Geometry check sheet. Reference: the model listing, model coordinates, mm. Round coordinates to 2 decimals unless told otherwise and drop trailing zeros. Write each loop counter-clockwise with the first axis right and the second up, starting at its lowest first coordinate (ties: lowest second). Pieces come first, ordered by that corner, then holes.
Item 1: Cross-section at A-A (x = -100). Enter the section's corners in (y, z).
Item 2: Draft check along X on faces 1 (the face through (-45, 2, 25)), 2 (the face through (150, 2, -1)), 3 (the face through (2, 5, -11)). Enter one of: pulls with the +X half, pulls with the -X half, needs draft (parallel to the pull), parting line crosses it, or undercut.
Item 3: Cross-section at C-C (x = 18). Enter the section's corners in (y, z), then the cut area to 3 significant figures.
Item 4: Cross-section at B-B (y = 3.05). State how many separate pieces and enclosed holes the cut face has, then the cut area to 3 significant figures.
Item 5: Scan lines: probe 1 along Z at (x, y) = (92, 1.8); probe 2 along Z at (x, y) = (138.25, 3.35); probe 3 along X at (y, z) = (0.9, -28). Record each from-to range of solid material in increasing order.
Item 6: Depth check by flat-ended pin: P1, Ø9, axis at x = 0, z = 0, coming from the +Y side. Enter the tip coordinate at first touch or a pass-through.
from build123d import *

# Parameters (mm, degrees)
SKETCH1_R           = 7.5
SKETCH1_R_2         = 1.75
SKETCH1_W           = 5
SKETCH1_H           = 10
BOSS_EXTRUDE2_DEPTH = 5


with BuildPart() as part:
    # Sketch1 → Boss-Extrude2 (new body)
    with BuildSketch(Plane(origin=(0, 0, 0), x_dir=(1, 0, 0), z_dir=(0, 1, 0))):
        Polygon((-50, 45), (150, 45), (150, -45), (-50, -45), (-150, -45), (-150, 45), align=None)
        Circle(SKETCH1_R, mode=Mode.SUBTRACT)
        with Locations((100, 0)):
            Circle(SKETCH1_R, mode=Mode.SUBTRACT)
        with Locations((-100, 0)):
            Circle(SKETCH1_R, mode=Mode.SUBTRACT)
        with Locations((-138.25, 25)):
            Circle(SKETCH1_R_2, mode=Mode.SUBTRACT)
        with Locations((-130, 38.25)):
            Circle(SKETCH1_R_2, mode=Mode.SUBTRACT)
        with Locations((-138.25, -25)):
            Circle(SKETCH1_R_2, mode=Mode.SUBTRACT)
        with Locations((-70, 38.25)):
            Circle(SKETCH1_R_2, mode=Mode.SUBTRACT)
        with Locations((-30, 38.25)):
            Circle(SKETCH1_R_2, mode=Mode.SUBTRACT)
        with Locations((30, 38.25)):
            Circle(SKETCH1_R_2, mode=Mode.SUBTRACT)
        with Locations((70, 38.25)):
            Circle(SKETCH1_R_2, mode=Mode.SUBTRACT)
        with Locations((130, 38.25)):
            Circle(SKETCH1_R_2, mode=Mode.SUBTRACT)
        with Locations((-130, -38.25)):
            Circle(SKETCH1_R_2, mode=Mode.SUBTRACT)
        with Locations((-70, -38.25)):
            Circle(SKETCH1_R_2, mode=Mode.SUBTRACT)
        with Locations((-30, -38.25)):
            Circle(SKETCH1_R_2, mode=Mode.SUBTRACT)
        with Locations((30, -38.25)):
            Circle(SKETCH1_R_2, mode=Mode.SUBTRACT)
        with Locations((70, -38.25)):
            Circle(SKETCH1_R_2, mode=Mode.SUBTRACT)
        with Locations((130, -38.25)):
            Circle(SKETCH1_R_2, mode=Mode.SUBTRACT)
        with Locations((138.25, -25)):
            Circle(SKETCH1_R_2, mode=Mode.SUBTRACT)
        with Locations((138.25, 25)):
            Circle(SKETCH1_R_2, mode=Mode.SUBTRACT)
        with BuildLine():
            Line((-21.910531466, 30), (21.910531466, 30))
            ThreePointArc((21.910531466, 30), (23.786301496, 28.693892495), (23.212114213, 26.481486795))
            Line((23.212114213, 26.481486795), (8.508395839, 13.878299617))
            ThreePointArc((8.508395839, 13.878299617), (7.476831919, 13.41512419), (6.358952728, 13.585423078))
            ThreePointArc((6.358952728, 13.585423078), (0, 15), (-6.358952728, 13.585423078))
            ThreePointArc((-6.358952728, 13.585423078), (-7.476831919, 13.41512419), (-8.508395839, 13.878299617))
            Line((-8.508395839, 13.878299617), (-23.212114213, 26.481486795))
            ThreePointArc((-23.212114213, 26.481486795), (-23.786301496, 28.693892495), (-21.910531466, 30))
        make_face(mode=Mode.SUBTRACT)
        with BuildLine():
            Line((-35, 19.066169828), (-35, -19.066169828))
            ThreePointArc((-35, -19.066169828), (-33.835713619, -20.883195625), (-31.698417253, -20.584683033))
            Line((-31.698417253, -20.584683033), (-15.016309573, -6.285733593))
            ThreePointArc((-15.016309573, -6.285733593), (-14.400814669, -5.337144314), (-14.398140282, -4.206370931))
            ThreePointArc((-14.398140282, -4.206370931), (-15, 0), (-14.398140282, 4.206370931))
            ThreePointArc((-14.398140282, 4.206370931), (-14.400814669, 5.337144314), (-15.016309573, 6.285733593))
            Line((-15.016309573, 6.285733593), (-31.698417253, 20.584683033))
            ThreePointArc((-31.698417253, 20.584683033), (-33.835713619, 20.883195625), (-35, 19.066169828))
        make_face(mode=Mode.SUBTRACT)
        with BuildLine():
            Line((-21.910531466, -30), (21.910531466, -30))
            ThreePointArc((21.910531466, -30), (23.786301496, -28.693892495), (23.212114213, -26.481486795))
            Line((23.212114213, -26.481486795), (8.508395839, -13.878299617))
            ThreePointArc((8.508395839, -13.878299617), (7.476831919, -13.41512419), (6.358952728, -13.585423078))
            ThreePointArc((6.358952728, -13.585423078), (0, -15), (-6.358952728, -13.585423078))
            ThreePointArc((-6.358952728, -13.585423078), (-7.476831919, -13.41512419), (-8.508395839, -13.878299617))
            Line((-8.508395839, -13.878299617), (-23.212114213, -26.481486795))
            ThreePointArc((-23.212114213, -26.481486795), (-23.786301496, -28.693892495), (-21.910531466, -30))
        make_face(mode=Mode.SUBTRACT)
        with BuildLine():
            Line((35, 19.066169828), (35, -19.066169828))
            ThreePointArc((35, -19.066169828), (33.835713619, -20.883195625), (31.698417253, -20.584683033))
            Line((31.698417253, -20.584683033), (15.016309573, -6.285733593))
            ThreePointArc((15.016309573, -6.285733593), (14.400814669, -5.337144314), (14.398140282, -4.206370931))
            ThreePointArc((14.398140282, -4.206370931), (15, 0), (14.398140282, 4.206370931))
            ThreePointArc((14.398140282, 4.206370931), (14.400814669, 5.337144314), (15.016309573, 6.285733593))
            Line((15.016309573, 6.285733593), (31.698417253, 20.584683033))
            ThreePointArc((31.698417253, 20.584683033), (33.835713619, 20.883195625), (35, 19.066169828))
        make_face(mode=Mode.SUBTRACT)
        with BuildLine():
            Line((131.698417253, -20.584683033), (115.016309573, -6.285733593))
            ThreePointArc((115.016309573, -6.285733593), (114.400814669, -5.337144314), (114.398140282, -4.206370931))
            ThreePointArc((114.398140282, -4.206370931), (115, 0), (114.398140282, 4.206370931))
            ThreePointArc((114.398140282, 4.206370931), (114.400814669, 5.337144314), (115.016309573, 6.285733593))
            Line((115.016309573, 6.285733593), (131.698417253, 20.584683033))
            ThreePointArc((131.698417253, 20.584683033), (133.835713619, 20.883195625), (135, 19.066169828))
            Line((135, 19.066169828), (135, -19.066169828))
            ThreePointArc((135, -19.066169828), (133.835713619, -20.883195625), (131.698417253, -20.584683033))
        make_face(mode=Mode.SUBTRACT)
        with BuildLine():
            Line((123.212114213, -26.481486795), (108.508395839, -13.878299617))
            ThreePointArc((108.508395839, -13.878299617), (107.476831919, -13.41512419), (106.358952728, -13.585423078))
            ThreePointArc((106.358952728, -13.585423078), (100, -15), (93.641047272, -13.585423078))
            ThreePointArc((93.641047272, -13.585423078), (92.523168081, -13.41512419), (91.491604161, -13.878299617))
            Line((91.491604161, -13.878299617), (76.787885787, -26.481486795))
            ThreePointArc((76.787885787, -26.481486795), (76.213698504, -28.693892495), (78.089468534, -30))
            Line((78.089468534, -30), (121.910531466, -30))
            ThreePointArc((121.910531466, -30), (123.786301496, -28.693892495), (123.212114213, -26.481486795))
        make_face(mode=Mode.SUBTRACT)
        with BuildLine():
            Line((68.301582747, -20.584683033), (84.983690427, -6.285733593))
            ThreePointArc((84.983690427, -6.285733593), (85.599185331, -5.337144314), (85.601859718, -4.206370931))
            ThreePointArc((85.601859718, -4.206370931), (85, 0), (85.601859718, 4.206370931))
            ThreePointArc((85.601859718, 4.206370931), (85.599185331, 5.337144314), (84.983690427, 6.285733593))
            Line((84.983690427, 6.285733593), (68.301582747, 20.584683033))
            ThreePointArc((68.301582747, 20.584683033), (66.164286381, 20.883195625), (65, 19.066169828))
            Line((65, 19.066169828), (65, -19.066169828))
            ThreePointArc((65, -19.066169828), (66.164286381, -20.883195625), (68.301582747, -20.584683033))
        make_face(mode=Mode.SUBTRACT)
        with BuildLine():
            Line((76.787885787, 26.481486795), (91.491604161, 13.878299617))
            ThreePointArc((91.491604161, 13.878299617), (92.523168081, 13.41512419), (93.641047272, 13.585423078))
            ThreePointArc((93.641047272, 13.585423078), (100, 15), (106.358952728, 13.585423078))
            ThreePointArc((106.358952728, 13.585423078), (107.476831919, 13.41512419), (108.508395839, 13.878299617))
            Line((108.508395839, 13.878299617), (123.212114213, 26.481486795))
            ThreePointArc((123.212114213, 26.481486795), (123.786301496, 28.693892495), (121.910531466, 30))
            Line((121.910531466, 30), (78.089468534, 30))
            ThreePointArc((78.089468534, 30), (76.213698504, 28.693892495), (76.787885787, 26.481486795))
        make_face(mode=Mode.SUBTRACT)
        with BuildLine():
            Line((-68.301582747, -20.584683033), (-84.983690427, -6.285733593))
            ThreePointArc((-84.983690427, -6.285733593), (-85.599185331, -5.337144314), (-85.601859718, -4.206370931))
            ThreePointArc((-85.601859718, -4.206370931), (-85, 0), (-85.601859718, 4.206370931))
            ThreePointArc((-85.601859718, 4.206370931), (-85.599185331, 5.337144314), (-84.983690427, 6.285733593))
            Line((-84.983690427, 6.285733593), (-68.301582747, 20.584683033))
            ThreePointArc((-68.301582747, 20.584683033), (-66.164286381, 20.883195625), (-65, 19.066169828))
            Line((-65, 19.066169828), (-65, -19.066169828))
            ThreePointArc((-65, -19.066169828), (-66.164286381, -20.883195625), (-68.301582747, -20.584683033))
        make_face(mode=Mode.SUBTRACT)
        with BuildLine():
            Line((-76.787885787, -26.481486795), (-91.491604161, -13.878299617))
            ThreePointArc((-91.491604161, -13.878299617), (-92.523168081, -13.41512419), (-93.641047272, -13.585423078))
            ThreePointArc((-93.641047272, -13.585423078), (-100, -15), (-106.358952728, -13.585423078))
            ThreePointArc((-106.358952728, -13.585423078), (-107.476831919, -13.41512419), (-108.508395839, -13.878299617))
            Line((-108.508395839, -13.878299617), (-123.212114213, -26.481486795))
            ThreePointArc((-123.212114213, -26.481486795), (-123.786301496, -28.693892495), (-121.910531466, -30))
            Line((-121.910531466, -30), (-78.089468534, -30))
            ThreePointArc((-78.089468534, -30), (-76.213698504, -28.693892495), (-76.787885787, -26.481486795))
        make_face(mode=Mode.SUBTRACT)
        with BuildLine():
            Line((-131.698417253, -20.584683033), (-115.016309573, -6.285733593))
            ThreePointArc((-115.016309573, -6.285733593), (-114.400814669, -5.337144314), (-114.398140282, -4.206370931))
            ThreePointArc((-114.398140282, -4.206370931), (-115, 0), (-114.398140282, 4.206370931))
            ThreePointArc((-114.398140282, 4.206370931), (-114.400814669, 5.337144314), (-115.016309573, 6.285733593))
            Line((-115.016309573, 6.285733593), (-131.698417253, 20.584683033))
            ThreePointArc((-131.698417253, 20.584683033), (-133.835713619, 20.883195625), (-135, 19.066169828))
            Line((-135, 19.066169828), (-135, -19.066169828))
            ThreePointArc((-135, -19.066169828), (-133.835713619, -20.883195625), (-131.698417253, -20.584683033))
        make_face(mode=Mode.SUBTRACT)
        with BuildLine():
            Line((-123.212114213, 26.481486795), (-108.508395839, 13.878299617))
            ThreePointArc((-108.508395839, 13.878299617), (-107.476831919, 13.41512419), (-106.358952728, 13.585423078))
            ThreePointArc((-106.358952728, 13.585423078), (-100, 15), (-93.641047272, 13.585423078))
            ThreePointArc((-93.641047272, 13.585423078), (-92.523168081, 13.41512419), (-91.491604161, 13.878299617))
            Line((-91.491604161, 13.878299617), (-76.787885787, 26.481486795))
            ThreePointArc((-76.787885787, 26.481486795), (-76.213698504, 28.693892495), (-78.089468534, 30))
            Line((-78.089468534, 30), (-121.910531466, 30))
            ThreePointArc((-121.910531466, 30), (-123.786301496, 28.693892495), (-123.212114213, 26.481486795))
        make_face(mode=Mode.SUBTRACT)
        with Locations((-47.5, 25)):
            Rectangle(SKETCH1_W, SKETCH1_H, mode=Mode.SUBTRACT)
        with Locations((-47.5, -25)):
            Rectangle(SKETCH1_W, SKETCH1_H, mode=Mode.SUBTRACT)
    extrude(amount=BOSS_EXTRUDE2_DEPTH)


solid = part.part
Resolved:
1. outline: (0, -45) - (5, -45) - (5, -30) - (0, -30) - close; (0, -15) - (5, -15) - (5, -7.5) - (0, -7.5) - close; (0, 7.5) - (5, 7.5) - (5, 15) - (0, 15) - close; (0, 30) - (5, 30) - (5, 45) - (0, 45) - close
2. face 1: undercut
2. face 2: pulls with the +X half
2. face 3: needs draft
3. outline: (0, -45) - (5, -45) - (5, -30) - (0, -30) - close; (0, -22.01) - (5, -22.01) - (5, -8.84) - (0, -8.84) - close; (0, 8.84) - (5, 8.84) - (5, 22.01) - (0, 22.01) - close; (0, 30) - (5, 30) - (5, 45) - (0, 45) - close
3. area: 282 mm2
4. separate pieces: 1
4. enclosed holes: 33
4. area: 19,300 mm2
5. probe 1: z = -45 to -30, -13.56 to 13.56, 30 to 45
5. probe 2: z = -45 to -26.75, -23.25 to 23.25, 26.75 to 45
5. probe 3: x = -150 to -123.91, -76.09 to -50, -45 to -23.91, 23.91 to 76.09, 123.91 to 150
6. P1: passes through
